Autodesk Fusion 360 part; units mm, degrees
sketch "Sketch1" plane through (0, 0, 0) normal (0, 1, 0) x (1, 0, 0)
  line L0 (14, -97.5) -> (14, -15.5) construction
  line L1 (14, -15.5) -> (96, -15.5) construction
  line L2 (96, -15.5) -> (96, -97.5) construction
  line L3 (96, -97.5) -> (14, -97.5) construction
  circle A0 centre (96, -15.5) radius 2
  circle A1 centre (14, -15.5) radius 2
  circle A2 centre (14, -97.5) radius 2
  circle A3 centre (96, -97.5) radius 2
  line L4 (0, 0) -> (110, 0)
  line L5 (110, 0) -> (110, -113)
  line L6 (110, -113) -> (0, -113)
  line L7 (0, -113) -> (0, 0)
  line L8 (101, -102.5) -> (9, -102.5)
  line L9 (9, -102.5) -> (9, -10.5)
  line L10 (9, -10.5) -> (101, -10.5)
  line L11 (101, -10.5) -> (101, -102.5)
  line L12 (55, -102.5) -> (55, -113) construction
  line L13 (101, -56.5) -> (110, -56.5) construction
  line L14 (94, -95.5) -> (16, -95.5)
  line L15 (16, -95.5) -> (16, -17.5)
  line L16 (16, -17.5) -> (94, -17.5)
  line L17 (94, -17.5) -> (94, -95.5)
  circle A4 centre (55, -56.5) radius 44.5
  line L18 (14, -97.5) -> (96, -15.5) construction
  line L19 (96, -97.5) -> (14, -15.5) construction
  point P0 (55, -97.5)
  point P1 (55, -102.5)
  point P2 (55, -113)
  point P3 (55, -56.5)
  dimension "d681" = 4
  dimension "d682" = 110
  dimension "d683" = 113
  dimension "d684" = 82
  dimension "d685" = 82
  dimension "d686" = -5
  dimension "d691" = 2
  dimension "d698" = 89
extrude "Extrude1" add sketch "Sketch1" along normal blind 20 contours L4 L5 L6 L7 | L8 L9 L10 L11 | L14 L17 A4 | L14 L15 A4 | L16 L17 A4 | L15 L16 A4
shell "Shell2" thickness 1.6 removed faces 1 at (56.1085, 20, 108.9585)
sketch "Sketch2" plane through (0, 20, 0) normal (0, 1, 0) x (-1, 0, 0)
  circle A0 centre (-96, 97.5) radius 2
  circle A1 centre (-14, 15.5) radius 2
  circle A2 centre (-96, 15.5) radius 2
  circle A3 centre (-14, 97.5) radius 2
  circle A4 centre (-96, 97.5) radius 3.6
  circle A5 centre (-14, 15.5) radius 3.6
  circle A6 centre (-14, 97.5) radius 3.6
  circle A7 centre (-96, 15.5) radius 3.6
  circle A8 centre (-55, 56.5) radius 46.1
  circle A9 centre (-55, 56.5) radius 44.5
  circle A10 centre (-55, 56.5) radius 46.1
extrude "Extrude3" cut sketch "Sketch2" against normal up to surface (20 mm away)
chamfer "Chamfer1" distance 2 angle 45 4 edges at (0, 10, 113) (110, 10, 113) (0, 10, 0) (110, 10, 0)
chamfer "Chamfer1" distance 2 angle 45 4 edges at (108.4, 10.8, 1.6) (1.6, 10.8, 1.6) (1.6, 10.8, 111.4) (108.4, 10.8, 111.4)
Check sheet for the modelled part. Datum: model origin and axes. Units: mm. A direction names the side the tool comes from. Round coordinates to 2 decimals unless told otherwise and drop trailing zeros. Write each loop counter-clockwise with the first axis right and the second up, starting at its lowest first coordinate (ties: lowest second). Pieces come first, ordered by that corner, then holes. Notation, with made-up numbers: (-24, 10.5) -> (35, 10.5) arc R24 ccw to (35, 39.5) -> close; hole circle Ø4 at (11.5, -6.5). An arc over 180 degrees is marked (long way). Put each result on its own line as item: value.
(1) Sectioned sample at D-D (z = 106). Enter the section's corners in (x, y).
Values found:
outline: (0, 0) -> (110, 0) -> (110, 20) -> (108.4, 20) -> (108.4, 1.6) -> (1.6, 1.6) -> (1.6, 20) -> (0, 20) -> close
(2) Go/stop test with a flat-tipped pin: pin 1 Ø11.5 at (x, z) = (96, 15.5) entering from +Y. Record where the tip stops, or that it passes through.
Values found:
pin 1: stops at y = 1.6
(3) Mould release check, pull along Z, two halves, no side actions. Record for faces 3 (the face through (56, 10, 113)), 4 (the face through (1.6, 11, 57)), 5 (the face through (110, 10, 56)): released by +Z, released by -Z, zero draft, split by the parting line, or undercut.
Values found:
face 3: released by +Z
face 4: undercut
face 5: zero draft
(4) Sectioned sample at A-A (y = 15.25). Enter the section's corners in (x, z), plus the area to 3 significant figures.
Values found:
outline: (0, 2) -> (2, 0) -> (108, 0) -> (110, 2) -> (110, 111) -> (108, 113) -> (2, 113) -> (0, 111) -> close; hole (1.6, 3.6) -> (3.6, 1.6) -> (106.4, 1.6) -> (108.4, 3.6) -> (108.4, 109.4) -> (106.4, 111.4) -> (3.6, 111.4) -> (1.6, 109.4) -> close
area: 703 mm^2
(5) Tool access check on faces 1 (the face through (0, 10, 57)), 2 (the face through (56, 11, 111.4)). Record the directions out of +Z, -Z, +X, -X, +Y, -Y that give a thin tool (end or side, any length) a straight path to the whole face; none if there is none.
Values found:
face 1: +Z, -Z, -X, +Y, -Y
face 2: +Y
(6) Sectioned sample at B-B (z = 56.5). Enter the section's corners in (x, y), plus the area to 3 significant figures.
Values found:
outline: (0, 0) -> (8.9, 0) -> (8.9, 1.6) -> (1.6, 1.6) -> (1.6, 20) -> (0, 20) -> close; (101.1, 0) -> (110, 0) -> (110, 20) -> (108.4, 20) -> (108.4, 1.6) -> (101.1, 1.6) -> close
area: 87.4 mm^2
(7) Material ranges on line 1 (X direction, y = 17, z = 104); line 2 (Z direction, x = 14, y = 0.95); line 3 (Z direction, x = 95, y = 17.5), recorded low to high.
Values found:
line 1: x = 0 to 1.6, 108.4 to 110
line 2: z = 0 to 11.9, 19.1 to 35.42, 77.58 to 93.9, 101.1 to 113
line 3: z = 0 to 1.6, 111.4 to 113
(8) Sectioned sample at C-C (x = 12.5). Enter the section's corners in (y, z).
Values found:
outline: (0, 0) -> (20, 0) -> (20, 1.6) -> (1.6, 1.6) -> (1.6, 12.23) -> (0, 12.23) -> close; (0, 18.77) -> (1.6, 18.77) -> (1.6, 38.64) -> (0, 38.64) -> close; (0, 74.36) -> (1.6, 74.36) -> (1.6, 94.23) -> (0, 94.23) -> close; (0, 100.77) -> (1.6, 100.77) -> (1.6, 111.4) -> (20, 111.4) -> (20, 113) -> (0, 113) -> close
